from build123d import *

# Parameters (mm, degrees)
SKETCH_1_W           = 300
SKETCH_1_H           = 300
EXTRUDE_1_DEPTH      = 7.5
SKETCH_2_W           = 80
SKETCH_2_H           = 50
CUT_EXTRUDE_1_DEPTH  = 50
SKETCH_3_R           = 1.6
SKETCH_3_R_2         = 1.600000001
SKETCH_3_R_3         = 1.599999999
CUT_EXTRUDE_2_DEPTH  = 500
CUT_EXTRUDE_4_DEPTH  = 0.01
SKETCH_6_W           = 140
SKETCH_6_H           = 5
CUT_EXTRUDE_5_DEPTH  = 400
SKETCH_7_W           = 140
SKETCH_7_H           = 5
CUT_EXTRUDE_6_DEPTH  = 500
SKETCH_8_W           = 2.5
SKETCH_8_H           = 200
CUT_EXTRUDE_7_DEPTH  = 500
SKETCH_9_W           = 2.5
SKETCH_9_H           = 200
CUT_EXTRUDE_8_DEPTH  = 500
FILLET_1_R           = 10
FILLET_2_R           = 10
FILLET_3_R           = 10
FILLET_4_R           = 10
FILLET_5_R           = 10
FILLET_6_R           = 10
SKETCH_11_R          = 1.5
CUT_EXTRUDE_9_DEPTH  = 500
SKETCH_12_R          = 1.5
CUT_EXTRUDE_10_DEPTH = 500
CUT_EXTRUDE_11_DEPTH = 50


with BuildPart() as part:
    # 草图1 → 凸台-拉伸1 (new body)
    with BuildSketch(Plane(origin=(0, 0, 0), x_dir=(1, 0, 0), z_dir=(0, 1, 0))):
        Rectangle(SKETCH_1_W, SKETCH_1_H)
    extrude(amount=EXTRUDE_1_DEPTH)

    # 草图2 → 切除-拉伸1 (cut)
    with BuildSketch(Plane(origin=(0, 0, 0), x_dir=(-1, 0, 0), z_dir=(0, -1, 0))):
        with Locations((-110, -125)):
            Rectangle(SKETCH_2_W, SKETCH_2_H)
        with Locations((-110, 125)):
            Rectangle(SKETCH_2_W, SKETCH_2_H)
        with Locations((110, -125)):
            Rectangle(SKETCH_2_W, SKETCH_2_H)
        with Locations((110, 125)):
            Rectangle(SKETCH_2_W, SKETCH_2_H)
    extrude(amount=-CUT_EXTRUDE_1_DEPTH, mode=Mode.SUBTRACT)

    # 草图3 → 切除-拉伸2 (cut)
    with BuildSketch(Plane.XZ):
        with Locations(Location((132.5, 81.505719169, 0), (0, 0, 270))):
            Circle(SKETCH_3_R)
        with Locations(Location((132.5, 57.505719169, 0), (0, 0, 270))):
            Circle(SKETCH_3_R)
        with Locations(Location((102.5, 81.505719169, 0), (0, 0, 270))):
            Circle(SKETCH_3_R)
        with Locations(Location((102.5, 57.505719169, 0), (0, 0, 270))):
            Circle(SKETCH_3_R)
        with Locations(Location((-102.5, 81.505719169, 0), (0, 0, 270))):
            Circle(SKETCH_3_R_2)
        with Locations(Location((-102.5, 57.505719169, 0), (0, 0, 270))):
            Circle(SKETCH_3_R_2)
        with Locations(Location((-132.5, 81.505719169, 0), (0, 0, 270))):
            Circle(SKETCH_3_R_2)
        with Locations(Location((-132.5, 57.505719169, 0), (0, 0, 270))):
            Circle(SKETCH_3_R_2)
        with Locations(Location((-132.5, -57.505719169, 0), (0, 0, 270))):
            Circle(SKETCH_3_R_3)
        with Locations(Location((-132.5, -81.505719169, 0), (0, 0, 270))):
            Circle(SKETCH_3_R_3)
        with Locations(Location((-102.5, -57.505719169, 0), (0, 0, 270))):
            Circle(SKETCH_3_R_3)
        with Locations(Location((-102.5, -81.505719169, 0), (0, 0, 270))):
            Circle(SKETCH_3_R_3)
        with Locations(Location((132.5, -81.505719169, 0), (0, 0, 270))):
            Circle(SKETCH_3_R)
        with Locations(Location((132.5, -57.505719169, 0), (0, 0, 270))):
            Circle(SKETCH_3_R)
        with Locations(Location((102.5, -57.505719169, 0), (0, 0, 270))):
            Circle(SKETCH_3_R)
        with Locations(Location((102.5, -81.505719169, 0), (0, 0, 270))):
            Circle(SKETCH_3_R)
    extrude(amount=-CUT_EXTRUDE_2_DEPTH, mode=Mode.SUBTRACT)

    # 草图5 → 切除-拉伸4 (cut)
    with BuildSketch(Plane.XZ):
        Polygon((145.77960396, 0), (141.689907669, 4.08969629), (141.689907669, -4.08969629), align=None)
    extrude(amount=-CUT_EXTRUDE_4_DEPTH, mode=Mode.SUBTRACT)

    # 草图6 → 切除-拉伸5 (cut)
    with BuildSketch(Plane(origin=(0, 7.5, 0), x_dir=(1, 0, 0), z_dir=(0, 1, 0))):
        with Locations((0, 147.5)):
            Rectangle(SKETCH_6_W, SKETCH_6_H)
    extrude(amount=-CUT_EXTRUDE_5_DEPTH, mode=Mode.SUBTRACT)

    # 草图7 → 切除-拉伸6 (cut)
    with BuildSketch(Plane(origin=(0, 7.5, 0), x_dir=(1, 0, 0), z_dir=(0, 1, 0))):
        with Locations((0, -147.5)):
            Rectangle(SKETCH_7_W, SKETCH_7_H)
    extrude(amount=-CUT_EXTRUDE_6_DEPTH, mode=Mode.SUBTRACT)

    # 草图8 → 切除-拉伸7 (cut)
    with BuildSketch(Plane(origin=(0, 7.5, 0), x_dir=(1, 0, 0), z_dir=(0, 1, 0))):
        with Locations((-148.75, 0)):
            Rectangle(SKETCH_8_W, SKETCH_8_H)
    extrude(amount=-CUT_EXTRUDE_7_DEPTH, mode=Mode.SUBTRACT)

    # 草图9 → 切除-拉伸8 (cut)
    with BuildSketch(Plane(origin=(0, 7.5, 0), x_dir=(1, 0, 0), z_dir=(0, 1, 0))):
        with Locations((148.75, 0)):
            Rectangle(SKETCH_9_W, SKETCH_9_H)
    extrude(amount=-CUT_EXTRUDE_8_DEPTH, mode=Mode.SUBTRACT)

    # 圆角1
    fillet_1_edges = [part.edges().sort_by_distance(p)[0] for p in [
        (-70, 3.75, 145),
        (70, 3.75, 145),
    ]]
    fillet(fillet_1_edges, radius=FILLET_1_R)

    # 圆角2
    fillet_2_edges = [part.edges().sort_by_distance(p)[0] for p in [
        (-70, 3.75, 100),
        (70, 3.75, 100),
    ]]
    fillet(fillet_2_edges, radius=FILLET_2_R)

    # 圆角3
    fillet_3_edges = [part.edges().sort_by_distance(p)[0] for p in [
        (-147.5, 3.75, 100),
        (147.5, 3.75, 100),
    ]]
    fillet(fillet_3_edges, radius=FILLET_3_R)

    # 圆角4
    fillet_4_edges = [part.edges().sort_by_distance(p)[0] for p in [
        (-147.5, 3.75, -100),
        (147.5, 3.75, -100),
    ]]
    fillet(fillet_4_edges, radius=FILLET_4_R)

    # 圆角5
    fillet_5_edges = [part.edges().sort_by_distance(p)[0] for p in [
        (70, 3.75, -100),
        (-70, 3.75, -100),
    ]]
    fillet(fillet_5_edges, radius=FILLET_5_R)

    # 圆角6
    fillet_6_edges = [part.edges().sort_by_distance(p)[0] for p in [
        (70, 3.75, -145),
        (-70, 3.75, -145),
    ]]
    fillet(fillet_6_edges, radius=FILLET_6_R)

    # 草图11 → 切除-拉伸9 (cut)
    with BuildSketch(Plane.XZ):
        with Locations(Location((-50, 125, 0), (0, 0, 270))):
            Circle(SKETCH_11_R)
    extrude(amount=-CUT_EXTRUDE_9_DEPTH, mode=Mode.SUBTRACT)

    # 草图12 → 切除-拉伸10 (cut)
    with BuildSketch(Plane.XZ):
        with Locations(Location((50, 125, 0), (0, 0, 270))):
            Circle(SKETCH_12_R)
        with Locations(Location((70, 80, 0), (0, 0, 270))):
            Circle(SKETCH_12_R)
        with Locations(Location((70, 0, 0), (0, 0, 270))):
            Circle(SKETCH_12_R)
        with Locations(Location((70, -80, 0), (0, 0, 270))):
            Circle(SKETCH_12_R)
        with Locations(Location((50, -125, 0), (0, 0, 270))):
            Circle(SKETCH_12_R)
        with Locations(Location((-50, -125, 0), (0, 0, 270))):
            Circle(SKETCH_12_R)
        with Locations(Location((-82.5, -85, 0), (0, 0, 270))):
            Circle(SKETCH_12_R)
        with Locations(Location((-132.5, 0, 0), (0, 0, 270))):
            Circle(SKETCH_12_R)
        with Locations(Location((-50, 125, 0), (0, 0, 270))):
            Circle(SKETCH_12_R)
        with Locations(Location((-82.5, 85, 0), (0, 0, 270))):
            Circle(SKETCH_12_R)
    extrude(amount=-CUT_EXTRUDE_10_DEPTH, mode=Mode.SUBTRACT)

    # 草图13 → 切除-拉伸11 (cut)
    with BuildSketch(Plane(origin=(0, 7.5, 0), x_dir=(1, 0, 0), z_dir=(0, 1, 0))):
        with BuildLine():
            Line((-10, -20), (-10, 20))
            ThreePointArc((-10, 20), (0, 30), (10, 20))
            Line((10, 20), (10, -20))
            ThreePointArc((10, -20), (0, -30), (-10, -20))
        make_face()
    extrude(amount=-CUT_EXTRUDE_11_DEPTH, mode=Mode.SUBTRACT)


solid = part.part
Could you check a few things on this model? Use its own coordinates, in mm. A direction names the side the tool comes from. Coordinates: 2 decimals unless noted, no trailing zeros. Order: outer loops, then holes, each group sorted by start corner. A loop starts at its lowest first (then second) coordinate and runs counter-clockwise, first axis right, second up. Notation, with made-up numbers: (46, 87) -> (51, 87) arc R31 cw to (51, 117) -> close; hole circle Ø6 at (18.25, 83). An arc over 180 degrees is marked (long way). One line per item, written item: value. Start each with the question number.
1) Imagine slicing it at A-A on z = -16.5. List the corners of the cut face in (x, y) for me, plus the area to 3 significant figures.
2) I'm going to push flat-ended pins straight in: pin 1 (3 mm diameter, centred on x = -102.5, z = -57.51, fed in from +Y); pin 2 (2 mm diameter, centred on y = 3, z = 111.5, fed in from +X); pin 3 (2 mm diameter, centred on y = 2, z = -126.5, fed in from -X). Where does each tip first touch, or does it pass through?
3) Imagine slicing it at B-B on x = 91.5. List the corners of the cut face in (y, z) for me.
4) If I drill on L1, parallel to X at y = 2.25, z = 125; L2, parallel to Z at x = 102.5, y = 1.75; L3, parallel to X at y = 6.5, z = 57.5, over which ranges is the centre line in solid material (lowest first)? Write a range as [from, to].
5) We'd pull the mould along Z, two halves only. Please class faces 1 (the cylindrical face through (-72.85, 3.8, 103.01)), 2 (the flat face through (-10, 4, 0)), 3 (the flat face through (-2, 0, -34)): +Z half, -Z half, draft (parallel to the pull), parting line (faces both ways), or undercut.
6) Imagine slicing it at C-C on y = 2.5. Count the separate pieces of the cut face and the enclosed holes in it, plus the area to 3 significant figures.
7) Which directions (+Z, -Z, +X, -X, +Y, -Y) give clear straight access to the entire face, cutting with the end or side of a thin tool? Please do faces 4 (the flat face through (70, 4, -122)), 5 (the flat face through (-70, 4, 123)), 6 (the cylindrical face through (0, 4, -30)), 7 (the flat face through (-1, 4, 145)), 8 (the flat face through (147.5, 4, 1)).
Answer list:
1. outline: (-147.5, 0) -> (-10, 0) -> (-10, 7.5) -> (-147.5, 7.5) -> close; (10, 0) -> (147.5, 0) -> (147.5, 7.5) -> (10, 7.5) -> close
1. area: 2,060 mm2
2. pin 1: passes through
2. pin 2: stops at x = 70
2. pin 3: stops at x = -70
3. outline: (0, -100) -> (7.5, -100) -> (7.5, 100) -> (0, 100) -> close
4. L1: x = [-70, -51.5], [-48.5, 48.5], [51.5, 70]
4. L2: z = [-100, -83.11], [-79.91, -59.11], [-55.91, 55.91], [59.11, 79.91], [83.11, 100]
4. L3: x = [-147.5, -134.1], [-130.9, -104.1], [-100.9, 100.9], [104.1, 130.9], [134.1, 147.5]
5. face 1: +Z half
5. face 2: undercut
5. face 3: draft
6. separate pieces: 1
6. enclosed holes: 27
6. area: 70,200 mm2
7. face 4: -Z, +X, +Y, -Y
7. face 5: +Z, -X, +Y, -Y
7. face 6: +Y, -Y
7. face 7: +Z, +X, -X, +Y, -Y
7. face 8: +Z, -Z, +X, +Y, -Y
